```python
from build123d import *

# Parameters (mm, degrees)
CYLINDER070_R     = 1.6
CYLINDER070_DEPTH = 2
BOX178_W          = 10
BOX178_H          = 2
BOX178_DEPTH      = 8
FILLET039_R       = 3
BOX180_W          = 2
BOX180_H          = 2
BOX180_DEPTH      = 1.5
BOX179_W          = 2
BOX179_H          = 2
BOX179_DEPTH      = 1.5


with BuildPart() as cylinder151:
    # Cylinder070 → Cylinder070 (new body)
    with BuildSketch(Plane(origin=(35, 33, -22), x_dir=(1, 0, 0), z_dir=(0, -1, 0))):
        Circle(CYLINDER070_R)
    extrude(amount=CYLINDER070_DEPTH)


with BuildPart() as fillet039:
    # Box178 → Box178 (new body)
    with BuildSketch(Plane(origin=(30, 31, -25), x_dir=(1, 0, 0), z_dir=(0, 0, 1))):
        with Locations((5, 1)):
            Rectangle(BOX178_W, BOX178_H)
    extrude(amount=BOX178_DEPTH)

    # Cut094: cut Cylinder151
    add(cylinder151.part, mode=Mode.SUBTRACT)

    # Fillet039
    fillet039_edges = [fillet039.edges().sort_by_distance(p)[0] for p in [
        (30, 32, -25),
        (40, 32, -25),
    ]]
    fillet(fillet039_edges, radius=FILLET039_R)


with BuildPart() as cube169:
    # Box180 → Box180 (new body)
    with BuildSketch(Plane(origin=(30, 29, -20.5), x_dir=(1, 0, 0), z_dir=(0, 0, 1))):
        with Locations((1, 1)):
            Rectangle(BOX180_W, BOX180_H)
    extrude(amount=BOX180_DEPTH)


with BuildPart() as fusion054:
    # Box179 → Box179 (new body)
    with BuildSketch(Plane(origin=(38, 29, -20.5), x_dir=(1, 0, 0), z_dir=(0, 0, 1))):
        with Locations((1, 1)):
            Rectangle(BOX179_W, BOX179_H)
    extrude(amount=BOX179_DEPTH)

    # Fusion054: union Fillet039, Cube169
    add(fillet039.part)
    add(cube169.part)


solid = fusion054.part
```
The model under review builds one solid part; all positions refer to its coordinate system, in mm. A direction names the side the tool comes from. Round coordinates to 2 decimals unless told otherwise and drop trailing zeros. Loops run counter-clockwise (first coordinate to the right, second up) from the corner with the lowest first, then second, coordinate; pieces in that order, holes last. Notation, with made-up numbers: M -16,27 L 26,27 A21 ccw 26,64 Z; hole C 50.25,-39 d2. An arc over 180 degrees is marked long. Put each result on its own line as item: value.
Q1. To check wall thickness, follow L1, parallel to Z at x = 35, y = 32.45; L2, parallel to X at y = 30.6, z = -20.25; L3, parallel to Y at x = 34, z = -17.25. State the ranges of each line that lie inside material, in increasing order.
Result set:
L1: z = -25 to -23.6, -20.4 to -17
L2: x = 30 to 32, 38 to 40
L3: y = 31 to 33
Q2. Consider section D-D, the plane z = -19.5. Give the boundary of the cut face in (x, y).
Result set:
outline: M 30,29 L 32,29 L 32,31 L 38,31 L 38,29 L 40,29 L 40,33 L 30,33 Z
Q3. For pin 1 (2.5 mm diameter, centred on x = 34, z = -21, fed in from -Y); pin 2 (0.6 mm diameter, centred on x = 38.5, y = 30, fed in from +Z); pin 3 (2 mm diameter, centred on x = 31.5, y = 30.5, fed in from -Z), all flat-tipped, find the tip position at first contact; note any pin that passes through.
Result set:
pin 1: stops at y = 31
pin 2: stops at z = -19
pin 3: stops at z = -24.93
Q4. Consider section A-A, the plane x = 35. Give the boundary of the cut face in (y, z).
Result set:
outline: M 31,-25 L 33,-25 L 33,-23.6 L 31,-23.6 Z; M 31,-20.4 L 33,-20.4 L 33,-17 L 31,-17 Z
Q5. Machinability: for faces 1 (the flat face through (32, 30, -20)), 2 (the flat face through (35, 32, -25)), 3 (the flat face through (31, 30, -20.5)), 4 (the flat face through (31, 30, -19)), 5 (the flat face through (30, 32, -20)), which of the approach directions +Z, -Z, +X, -X, +Y, -Y give a long, thin tool a straight path to every point of the face, cutting with its end or side? Answer none if there is none.
Result set:
face 1: +Z, -Z, -Y
face 2: -Z, +X, -X, +Y, -Y
face 3: -Z, +X, -X, -Y
face 4: +Z, +X, -X, -Y
face 5: +Z, -Z, -X, +Y, -Y
Q6. Mouldability with a two-part tool opening along Z and no side actions: class faces 6 (the flat face through (39, 30, -19)), 7 (the cylindrical face through (30.86, 32.01, -24.1)), 8 (the cylindrical face through (33.82, 32.01, -20.92)) as released by +Z, released by -Z, zero draft, split by the parting line, or undercut.
Result set:
face 6: released by +Z
face 7: released by -Z
face 8: undercut
Q7. Consider section B-B, the plane y = 30.1. Give the boundary of the cut face in (x, z).
Result set:
outline: M 30,-20.5 L 32,-20.5 L 32,-19 L 30,-19 Z; M 38,-20.5 L 40,-20.5 L 40,-19 L 38,-19 Z
Q8. Consider section C-C, the plane y = 32.5. Give the boundary of the cut face in (x, z).
Result set:
outline: M 30,-22 A3 ccw 33,-25 L 37,-25 A3 ccw 40,-22 L 40,-17 L 30,-17 Z; hole C 35,-22 d3.2
